Here's the drawing with two shaded views (mm, measured from the low corner). I have some questions. Coordinates: 2 decimals unless noted, no trailing zeros. Write each loop counter-clockwise with the first axis right and the second up, starting at its lowest first coordinate (ties: lowest second). Pieces come first, ordered by that corner, then holes. Notation, with made-up numbers: (44.25, 7.5) -> (81.25, 7.5) arc R13 cw to (81.25, 15.5) -> close; hole circle Ø11 at (21.25, 33). An arc over 180 degrees is marked (long way). Use one line per item in the form item = value.
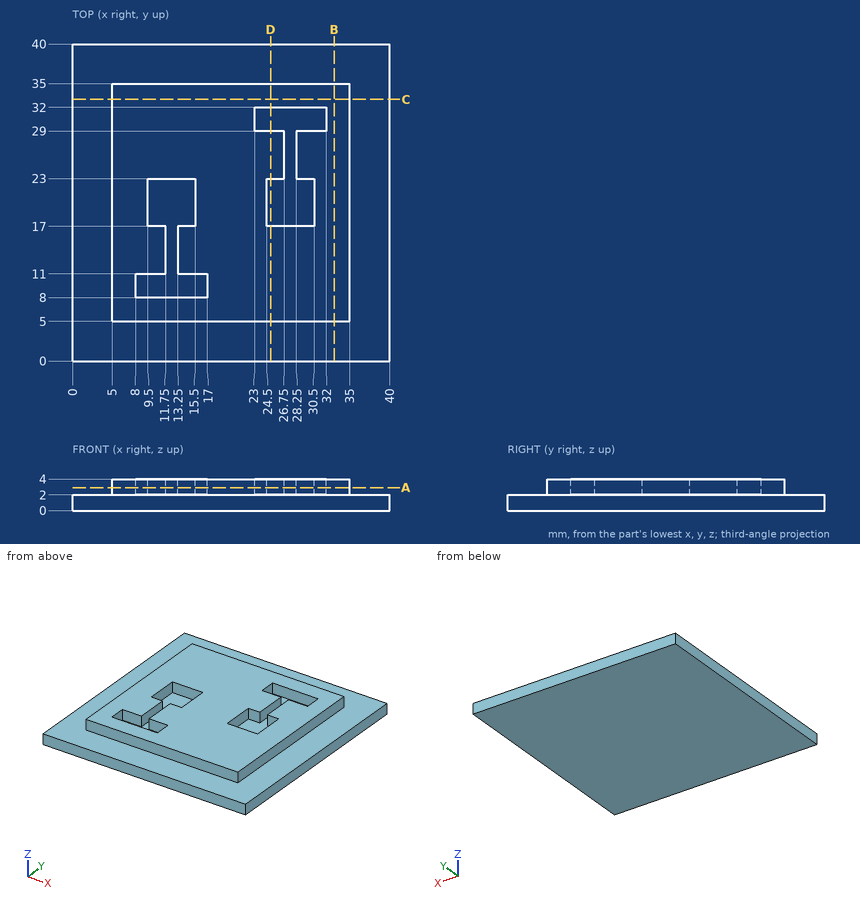
Q1. Will these pins go through, and if not, where does the flat tip stop? pin 1 (1 mm diameter, centred on x = 12.5, z = 3, fed in from +Y); pin 2 (0.6 mm diameter, centred on y = 19.5, z = 3, fed in from +X); pin 3 (0.6 mm diameter, centred on y = 19.5, z = 2.5, fed in from -X).
Return value:
pin_1 = 35
pin_2 = 35
pin_3 = 5
Q2. Suppose I cut it at B-B (x = 33). Write out the boundary of the cut face in (y, z).
Return value:
outline = (0, 0) -> (40, 0) -> (40, 2) -> (35, 2) -> (35, 4) -> (5, 4) -> (5, 2) -> (0, 2) -> close
Q3. Suppose I cut it at D-D (x = 25). Write out the boundary of the cut face in (y, z).
Return value:
outline = (0, 0) -> (40, 0) -> (40, 2) -> (35, 2) -> (35, 4) -> (32, 4) -> (32, 2) -> (29, 2) -> (29, 4) -> (23, 4) -> (23, 2) -> (17, 2) -> (17, 4) -> (5, 4) -> (5, 2) -> (0, 2) -> close
Q4. If I drill on line 1 (X direction, y = 17.5, z = 2.55); line 2 (Y direction, x = 16, z = 2.35); line 3 (X direction, y = 9, z = 3.7), over which ranges is the centre line in solid material (lowest first)? Write a range as from..to.
Return value:
line_1 = 5..9.5, 15.5..24.5, 30.5..35
line_2 = 5..8, 11..35
line_3 = 5..8, 17..35
Q5. Suppose I cut it at A-A (z = 2.9). Write out the boundary of the cut face in (x, y), then the cut area to 3 significant figures.
Return value:
outline = (5, 5) -> (35, 5) -> (35, 35) -> (5, 35) -> close; hole (8, 8) -> (17, 8) -> (17, 11) -> (13.25, 11) -> (13.25, 17) -> (15.5, 17) -> (15.5, 23) -> (9.5, 23) -> (9.5, 17) -> (11.75, 17) -> (11.75, 11) -> (8, 11) -> close; hole (23, 29) -> (26.75, 29) -> (26.75, 23) -> (24.5, 23) -> (24.5, 17) -> (30.5, 17) -> (30.5, 23) -> (28.25, 23) -> (28.25, 29) -> (32, 29) -> (32, 32) -> (23, 32) -> close
area = 756 mm2
